Check sheet for the drawn part. Datum: minimum x, y, z corner. Units: mm. A direction names the side the tool comes from. Coordinates: 2 decimals unless noted, no trailing zeros. Write each loop counter-clockwise with the first axis right and the second up, starting at its lowest first coordinate (ties: lowest second). Pieces come first, ordered by that corner, then holes. Notation, with made-up numbers: (20, 58) -> (36, 58) arc R14 cw to (36, 83) -> close; hole circle Ø1 at (34.5, 57.25). An arc over 180 degrees is marked (long way). Answer in a Markdown table with one row per item. Add a question column.
1. Cross-section at C-C on z = 13. Record the cut outline in (x, y), and give its area (4 significant figures).
2. Set-up check for the marked faces 1, 2, 3 and 4: record each of +Z, -Z, +X, -X, +Y, -Y from which the full face is reachable in a straight line by a thin tool's end or side.
3. Cross-section at B-B on x = 20. Record the cut outline in (y, z), and give its area (3 significant figures).
4. Cross-section at D-D on x = 114. Record the cut outline in (y, z).
5. Scan lines: L1, parallel to Y at x = 20, z = 37; L2, parallel to Y at x = 230, z = 37.3; L3, parallel to X at y = 156, z = 25.5. Record each from-to range of solid material in increasing order. Write a range as from..to.
6. Cross-section at A-A on y = 180. Record the cut outline in (x, z).
7. Depth check by flat-ended pin: P1, Ø10, axis at x = 118.5, z = 29.5, coming from the +Y side; P2, Ø2.5, axis at x = 37.5, z = 25, coming from the -Y side; P3, Ø2.5, axis at y = 163, z = 20, coming from the +X side. Enter the tip coordinate at first touch or a pass-through.
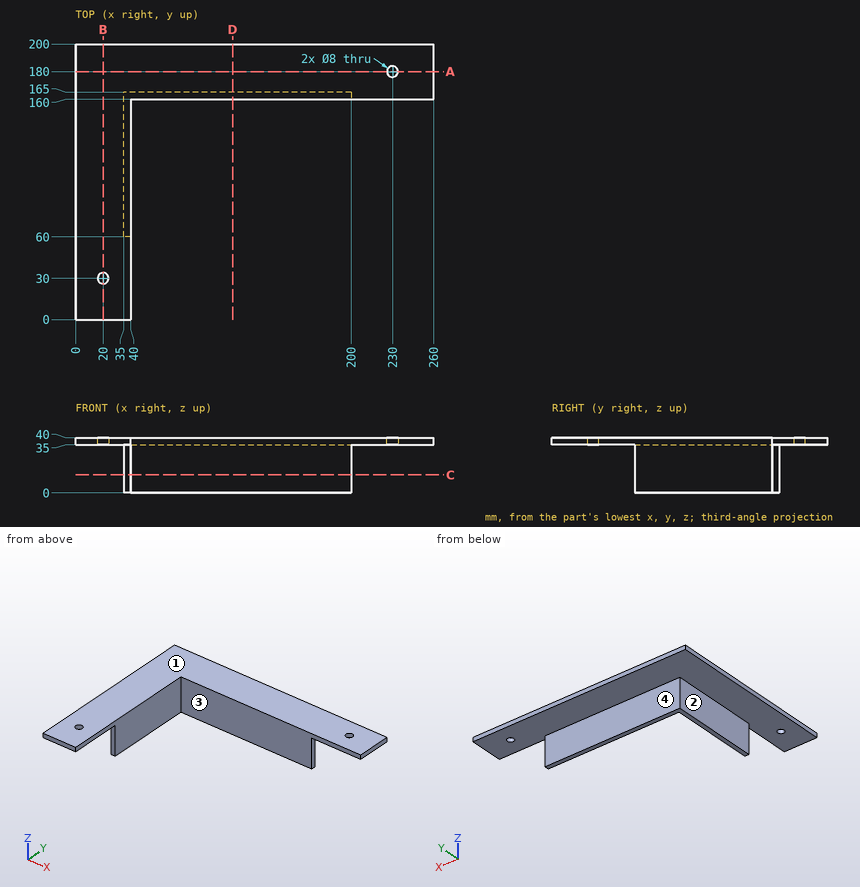
Results found:
| question | item | result |
|---|---|---|
| 1 | outline | (35, 60) -> (40, 60) -> (40, 160) -> (200, 160) -> (200, 165) -> (35, 165) -> close |
| 1 | area | 1,325 mm^2 |
| 2 | face 1 | +Z, +X, -X, +Y, -Y |
| 2 | face 2 | -Z, -X, +Y, -Y |
| 2 | face 3 | +Z, -Z, +X, -Y |
| 2 | face 4 | -Z, +X, -X, +Y |
| 3 | outline | (0, 35) -> (26, 35) -> (26, 40) -> (0, 40) -> close; (34, 35) -> (200, 35) -> (200, 40) -> (34, 40) -> close |
| 3 | area | 960 mm^2 |
| 4 | outline | (160, 0) -> (165, 0) -> (165, 35) -> (200, 35) -> (200, 40) -> (160, 40) -> close |
| 5 | L1 | y = 0..26, 34..200 |
| 5 | L2 | y = 160..176, 184..200 |
| 5 | L3 | x = 35..40 |
| 6 | outline | (0, 35) -> (226, 35) -> (226, 40) -> (0, 40) -> close; (234, 35) -> (260, 35) -> (260, 40) -> (234, 40) -> close |
| 7 | P1 | stops at y = 165 |
| 7 | P2 | stops at y = 60 |
| 7 | P3 | stops at x = 200 |
